Geometry: final body of the model. Coordinates: model frame, mm. Round coordinates to 2 decimals unless told otherwise and drop trailing zeros. Write each loop counter-clockwise with the first axis right and the second up, starting at its lowest first coordinate (ties: lowest second). Pieces come first, ordered by that corner, then holes. Notation, with made-up numbers: (-18.75, -26) -> (22.25, -26) arc R32 ccw to (22.25, 2) -> close; hole circle Ø2 at (-11, 49). An arc over 180 degrees is marked (long way). One line per item, written item: value. Start each with the question number.
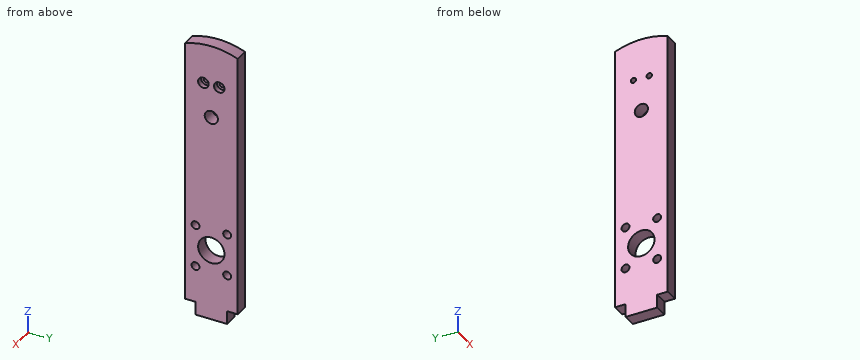
from build123d import *

# Parameters (mm, degrees)
F0_R           = 50
F0_R_2         = 25
F1_DEPTH       = 50
F2_D           = 30
F3_D           = 20
F3_CBORE_D     = 40
F3_CBORE_DEPTH = 20


with BuildPart() as f1:
    # F0 (on Right) → F1 (new body)
    with BuildSketch(Plane.YZ):
        with BuildLine():
            Line((-60, -25), (60, -25))
            Line((60, -25), (60, 25))
            Line((60, 25), (100, 25))
            Line((100, 25), (100, 1025))
            ThreePointArc((100, 1025), (0, 1043.567766), (-100, 1025))
            Line((-100, 1025), (-100, 25))
            Line((-100, 25), (-60, 25))
            Line((-60, 25), (-60, -25))
        make_face()
        with Locations((0, 245)):
            Circle(F0_R, mode=Mode.SUBTRACT)
        with Locations((0, 765)):
            Circle(F0_R_2, mode=Mode.SUBTRACT)
    extrude(amount=-F1_DEPTH)

    # F2 (through all)
    with Locations(Plane.YZ):
        with Locations((-60, 165), (-60, 325), (60, 325), (60, 165)):
            Hole(F2_D / 2)

    # F3 (through all)
    with Locations(Plane.YZ):
        with Locations((30, 891.491106), (-30, 891.491106)):
            CounterBoreHole(F3_D / 2, F3_CBORE_D / 2, F3_CBORE_DEPTH)


solid = f1.part
(1) Section query A-A (z = 245). Output: boundary loops of the cut face in (x, y).
(2) Section query C-C (z = 765). Output: boundary loops of the cut face in (x, y), and give its area (3 significant figures).
(3) Line query: probe 1 along Z at (x, y) = (-30, 0); probe 2 along Z at (x, y) = (-48, -56.5); probe 3 along Y at (x, z) = (-16, 335.5). Output: solid intervals per line, ascending.
(4) Section query D-D (y = -86.5). Output: boundary loops of the cut face in (x, z), and give its area (3 significant figures).
(5) Pin query (flat end, axial travel): pin 1 (24 mm diameter, centred on y = -30, z = 891.49, fed in from -X); pin 2 (10 mm diameter, centred on y = -30, z = 900, fed in from +X); pin 3 (15 mm diameter, centred on x = -23.5, z = -9.5, fed in from -Y); pin 4 (5 mm diameter, centred on x = -18.5, y = 31, fed in from +Z). Return the tip coordinate at first contact, or that it passes through.
(6) Section query B-B (x = -37). Count the separate pieces of the cut face and the enclosed holes in it, and give its area (3 significant figures).
Results list:
1. outline: (-50, -100) -> (0, -100) -> (0, -50) -> (-50, -50) -> close; (-50, 50) -> (0, 50) -> (0, 100) -> (-50, 100) -> close
2. outline: (-50, -100) -> (0, -100) -> (0, -25) -> (-50, -25) -> close; (-50, 25) -> (0, 25) -> (0, 100) -> (-50, 100) -> close
2. area: 7,500 mm^2
3. probe 1: z = -25 to 195, 295 to 740, 790 to 1043.57
3. probe 2: z = -25 to 150.41, 179.59 to 310.41, 339.59 to 1037.78
3. probe 3: y = -100 to -70.71, -49.29 to 49.29, 70.71 to 100
4. outline: (-50, 25) -> (0, 25) -> (0, 1029.8) -> (-50, 1029.8) -> close
4. area: 50,200 mm^2
5. pin 1: stops at x = -50
5. pin 2: stops at x = -20
5. pin 3: stops at y = -60
5. pin 4: stops at z = 1042.11
6. separate pieces: 1
6. enclosed holes: 8
6. area: 195,000 mm^2
